```python
from build123d import *

# Parameters (mm, degrees)
SKETCH1_W                    = 615
SKETCH1_H                    = 105
BASE_FLANGE1_DEPTH           = 0.75
EDGE_FLANGE1_STRIP_W         = 5
EDGE_FLANGE1_STRIP_H         = 0.75
EDGE_FLANGE1_STRIP_CUT_DEPTH = 615
EDGE_FLANGE1_DEPTH           = 615
SKETCH16_W                   = 615
SKETCH16_H                   = 196.52545168
CUT_EXTRUDE1_DEPTH           = 10
SWEPT_START                  = -307.5
SWEPT_FLANGE1_DEPTH          = 615
EDGE_FLANGE2_DEPTH           = 84
EDGE_FLANGE2_BEND_DEPTH      = 84
CUT_EXTRUDE2_DEPTH           = 623.102383053
CUT_EXTRUDE2_DEPTH_BACK      = 623.102383053
SKETCH39_R                   = 2.5
FILLET1_R                    = 8
SKETCH40_R                   = 1.5
CUT_EXTRUDE3_DEPTH           = 10


# Read off the part's stored shape, not the designer's step: Swept Flange1
# Sheet-metal steps are written as plain solids
with BuildPart() as part:
    # Sketch1 → Base-Flange1 (new body)
    with BuildSketch(Plane(origin=(0, 0, 0), x_dir=(1, 0, 0), z_dir=(0, 1, 0))):
        Rectangle(SKETCH1_W, SKETCH1_H)
    extrude(amount=-BASE_FLANGE1_DEPTH)

    # Edge-Flange1 strip (across the edge) → Edge-Flange1 strip cut (cut)
    with BuildSketch(Plane(origin=(307.5, -0.75, 52.5), x_dir=(0, 0, -1), z_dir=(-1, 0, 0))):
        with Locations((-1.5, -0.375)):
            Rectangle(EDGE_FLANGE1_STRIP_W, EDGE_FLANGE1_STRIP_H)
    extrude(amount=EDGE_FLANGE1_STRIP_CUT_DEPTH, mode=Mode.SUBTRACT)

    # Edge-Flange1 section (across the edge) → Edge-Flange1 (add)
    with BuildSketch(Plane(origin=(307.5, -0.75, 52.5), x_dir=(0, 0, -1), z_dir=(-1, 0, 0))):
        with BuildLine():
            Line((-0.75, 1), (-0.75, 7))
            Line((-0.75, 7), (0, 7))
            Line((0, 7), (0, 1))
            ThreePointArc((0, 1), (0.292893219, 0.292893219), (1, 0))
            Line((1, 0), (1, -0.75))
            ThreePointArc((1, -0.75), (-0.237436867, -0.237436867), (-0.75, 1))
        make_face()
    extrude(amount=EDGE_FLANGE1_DEPTH)

    # Sketch16 → Cut-Extrude1 (cut)
    with BuildSketch(Plane(origin=(0, 0, 0), x_dir=(1, 0, 0), z_dir=(0, 1, 0))):
        with Locations((0, 130.76272584)):
            Rectangle(SKETCH16_W, SKETCH16_H)
    extrude(amount=-CUT_EXTRUDE1_DEPTH, mode=Mode.SUBTRACT)

    # Swept Flange1 outline → Swept Flange1 (add)
    with BuildSketch(Plane.YZ.offset(SWEPT_START)):
        with BuildLine():
            Line((-1.7, -50.834586207), (-1.7, -53.75))
            Line((-1.7, -53.75), (-0.95, -53.75))
            Line((-0.95, -53.75), (-0.95, -50.834586207))
            ThreePointArc((-0.95, -50.834586207), (-1.097642895, -49.792701719), (-1.528945753, -48.832858214))
            Line((-1.528945753, -48.832858214), (-4.896680845, -43.497832325))
            ThreePointArc((-4.896680845, -43.497832325), (-5.357412506, -41.775852388), (-4.759837447, -40.09644993))
            Line((-4.759837447, -40.09644993), (-0.75, -34.75))
            ThreePointArc((-0.75, -34.75), (-0.192437632, -33.685854123), (0, -32.5))
            Line((0, -32.5), (-0.75, -32.5))
            ThreePointArc((-0.75, -32.5), (-0.903950106, -33.448683298), (-1.35, -34.3))
            Line((-1.35, -34.3), (-5.359837447, -39.64644993))
            ThreePointArc((-5.359837447, -39.64644993), (-6.106806271, -41.745703002), (-5.530891695, -43.898177923))
            Line((-5.530891695, -43.898177923), (-2.163156602, -49.233203812))
            ThreePointArc((-2.163156602, -49.233203812), (-1.818114316, -50.001078617), (-1.7, -50.834586207))
        make_face()
    extrude(amount=SWEPT_FLANGE1_DEPTH)

    # Edge-Flange2 section (across the edge) → Edge-Flange2 (add)
    with BuildSketch(Plane(origin=(308.5, -0.75, -32.5), x_dir=(-1, 0, 0), z_dir=(0, 0, 1))):
        with BuildLine():
            Line((-0.75, 1), (-0.75, 39))
            Line((-0.75, 39), (0, 39))
            Line((0, 39), (0, 1))
            ThreePointArc((0, 1), (0.292893219, 0.292893219), (1, 0))
            Line((1, 0), (1, -0.75))
            ThreePointArc((1, -0.75), (-0.237436867, -0.237436867), (-0.75, 1))
        make_face()
    extrude(amount=EDGE_FLANGE2_DEPTH)

    # Edge-Flange2 section 2 (across the edge) → Edge-Flange2 bend (add)
    with BuildSketch(Plane(origin=(-308.5, -0.75, 51.5), x_dir=(1, 0, 0), z_dir=(0, 0, -1))):
        with BuildLine():
            Line((-0.75, 1), (-0.75, 39))
            Line((-0.75, 39), (0, 39))
            Line((0, 39), (0, 1))
            ThreePointArc((0, 1), (0.292893219, 0.292893219), (1, 0))
            Line((1, 0), (1, -0.75))
            ThreePointArc((1, -0.75), (-0.237436867, -0.237436867), (-0.75, 1))
        make_face()
    extrude(amount=EDGE_FLANGE2_BEND_DEPTH)

    # Sketch39 → Cut-Extrude2 (cut, two sides: drawn at the far end of the back side and taken through both)
    with BuildSketch(Plane.ZY.offset(309.25).offset(-CUT_EXTRUDE2_DEPTH_BACK)):
        with Locations(Location((40, -32.5, 0), (0, 0, 90))):
            Circle(SKETCH39_R)
        with BuildLine():
            Line((-32.5, -10), (20.187006795, -10))
            Line((20.187006795, -10), (34.931706284, -36.756092926))
            ThreePointArc((34.931706284, -36.756092926), (37.056741569, -38.945618932), (40, -39.75))
            ThreePointArc((40, -39.75), (43.515434794, -38.559838948), (45.58487621, -35.47890121))
            Line((45.58487621, -35.47890121), (51.5, -13.685469847))
            Line((51.5, -13.685469847), (60.41713226, -13.685469847))
            Line((60.41713226, -13.685469847), (60.41713226, -59.649041705))
            Line((60.41713226, -59.649041705), (-51.871278106, -59.649041705))
            Line((-51.871278106, -59.649041705), (-51.871278106, -10))
            Line((-51.871278106, -10), (-32.5, -10))
        make_face()
    extrude(amount=CUT_EXTRUDE2_DEPTH + CUT_EXTRUDE2_DEPTH_BACK, mode=Mode.SUBTRACT)

    # Fillet1
    fillet1_edges = [part.edges().sort_by_distance(p)[0] for p in [
        (308.875, -10, -32.5),
        (-308.875, -10, -32.5),
    ]]
    fillet(fillet1_edges, radius=FILLET1_R)

    # Sketch40 → Cut-Extrude3 (cut)
    with BuildSketch(Plane(origin=(0, -23.135666601, -14.604389542), x_dir=(1, 0, 0), z_dir=(0, 0.8456144659552722, 0.5337941316342656))):
        with Locations(Location((0, 37.3231029, 0), (0, 0, 270))):
            Circle(SKETCH40_R)
    extrude(amount=-CUT_EXTRUDE3_DEPTH, mode=Mode.SUBTRACT)


solid = part.part
```
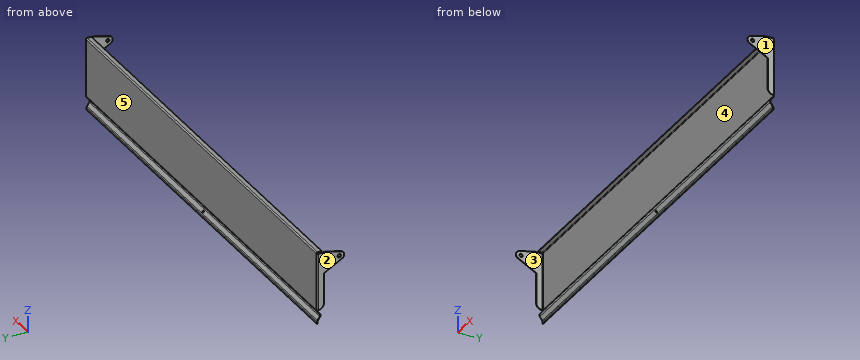
Check sheet for the modelled part. Datum: model origin and axes. Units: mm. Face numbers are marked on the shaded views. A direction names the side the tool comes from. Give positions to 0.01 mm unless a question says otherwise; leave off trailing zeros. Loops run counter-clockwise (first coordinate to the right, second up) from the corner with the lowest first, then second, coordinate; pieces in that order, holes last. Notation, with made-up numbers: (71, -17) - (125, -17) arc R25 cw to (125, 10) - close; hole circle Ø6 at (-18.5, -15). An arc over 180 degrees is marked (long way). One line per question, with ' | ' between items. Start each with the question number.
1. Cross-section at C-C, the plane z = -2. Enter the section's corners in (x, y).
2. Cross-section at A-A, the plane y = -22. Enter the section's corners in (x, z), plus the area to 3 significant figures.
3. Set-up check for the marked faces 4 and 5: record each of +Z, -Z, +X, -X, +Y, -Y from which the full face is reachable in a straight line by a thin tool's end or side.
4. Cross-section at B-B, the plane x = -239.5. Enter the section's corners in (y, z), plus the area to 3 significant figures.
5. Draft check along X on the marked faces 1, 2 and 3. Enter one of: released by +X, released by -X, zero draft, split by the parting line, or undercut.
6. Material ranges on line 1 along X through (y, z) = (-7, 47.5); line 2 along Z through (x, y) = (87.5, -3.5); line 3 along Y through (x, z) = (308, 40), recorded low to high. Write a range as [from, to].
7. Gauge pin test, flat ends, axial feed: pin 1 Ø0.9 at (x, z) = (-23, -52) entering from +Y; pin 2 Ø2.5 at (x, z) = (-47.5, -52.5) entering from -Y; pin 3 Ø1 at (x, z) = (164.5, -10) entering from -Y. Record the tip position at first contact, or that the pin passes through.
Check result:
1) outline: (-309.25, -10) - (-308.5, -10) - (-308.5, -1.75) arc R1 cw to (-307.5, -0.75) - (307.5, -0.75) arc R1 cw to (308.5, -1.75) - (308.5, -10) - (309.25, -10) - (309.25, -1.75) arc R1.75 ccw to (307.5, 0) - (-307.5, 0) arc R1.75 ccw to (-309.25, -1.75) - close
2) outline: (-309.25, 26.8) - (-308.5, 26.8) - (-308.5, 49.24) - (-309.25, 49.24) - close; (308.5, 26.8) - (309.25, 26.8) - (309.25, 49.24) - (308.5, 49.24) - close | area: 33.7 mm2
3) face 4: -Y | face 5: +Z, -Z, +X, -X, +Y
4) outline: (-7.75, 52.5) - (-1.75, 52.5) arc R1 cw to (-0.75, 51.5) - (-0.75, -32.5) arc R3 cw to (-1.35, -34.3) - (-5.36, -39.65) arc R3.75 ccw to (-5.53, -43.9) - (-2.16, -49.23) arc R3 cw to (-1.7, -50.83) - (-1.7, -53.75) - (-0.95, -53.75) - (-0.95, -50.83) arc R3.75 ccw to (-1.53, -48.83) - (-4.9, -43.5) arc R3 cw to (-4.76, -40.1) - (-0.75, -34.75) arc R3.75 ccw to (0, -32.5) - (0, 51.5) arc R1.75 ccw to (-1.75, 53.25) - (-7.75, 53.25) - close | area: 87.2 mm2
5) face 1: released by +X | face 2: released by -X | face 3: undercut
6) line 1: x = [-309.25, -308.5], [308.5, 309.25] | line 2: z = [-47.12, -45.71], [-38.42, -37.17], [52.5, 53.25] | line 3: y = [-0.88, -0.07]
7) pin 1: stops at y = -0.95 | pin 2: stops at y = -1.7 | pin 3: stops at y = -0.75
